from build123d import *

# Parameters (mm, degrees)
SKETCH1_W           = 22
SKETCH1_H           = 26
BOSS_EXTRUDE1_DEPTH = 40
SKETCH2_W           = 18.5
SKETCH2_H           = 22.5
CUT_EXTRUDE1_DEPTH  = 37
CUT_EXTRUDE2_REACH  = 54.536
CUT_EXTRUDE3_DEPTH  = 2
CUT_EXTRUDE4_START  = -1.5
CUT_EXTRUDE4_DEPTH  = 1.5
CUT_EXTRUDE5_REACH  = 54.536
CUT_EXTRUDE6_REACH  = 54.536
SKETCH12_R          = 2.3
BOSS_EXTRUDE2_DEPTH = 7.76
SKETCH14_R          = 1.65
CUT_EXTRUDE9_DEPTH  = 7.76
SKETCH16_R          = 1.65
CUT_EXTRUDE11_DEPTH = 7.76
BOSS_EXTRUDE3_START = 7.76
SKETCH17_R          = 2.3
BOSS_EXTRUDE3_DEPTH = 7.76
CUT_EXTRUDE12_START = -7.76
SKETCH20_R          = 1.65
CUT_EXTRUDE12_DEPTH = 7.76


with BuildPart() as part:
    # Sketch1 → Boss-Extrude1 (new body)
    with BuildSketch(Plane.XY):
        with Locations((11, 13)):
            Rectangle(SKETCH1_W, SKETCH1_H)
    extrude(amount=BOSS_EXTRUDE1_DEPTH)

    # Sketch2 → Cut-Extrude1 (cut)
    with BuildSketch(Plane.XY.offset(40)):
        with Locations((10.75, 13.25)):
            Rectangle(SKETCH2_W, SKETCH2_H)
    extrude(amount=-CUT_EXTRUDE1_DEPTH, mode=Mode.SUBTRACT)

    # Sketch6 → Cut-Extrude2 (cut, up to next)
    with BuildSketch(Plane(origin=(0, 0, 0), x_dir=(-1, 0, 0), z_dir=(0, 0, -1)), mode=Mode.PRIVATE) as cut_extrude2_sk1:
        with BuildLine():
            Line((-15, 22), (-7, 22))
            ThreePointArc((-7, 22), (-3.464466094, 20.535533906), (-2, 17))
            Line((-2, 17), (-2, 9))
            ThreePointArc((-2, 9), (-3.464466094, 5.464466094), (-7, 4))
            Line((-7, 4), (-15, 4))
            ThreePointArc((-15, 4), (-18.535533906, 5.464466094), (-20, 9))
            Line((-20, 9), (-20, 17))
            ThreePointArc((-20, 17), (-18.535533906, 20.535533906), (-15, 22))
        make_face()
    cut_extrude2_tool1 = extrude(cut_extrude2_sk1.sketch, amount=-CUT_EXTRUDE2_REACH, mode=Mode.PRIVATE) & part.part
    add(cut_extrude2_tool1.solids().sort_by_distance((11, 13, 0))[0], mode=Mode.SUBTRACT)

    # Sketch7 → Cut-Extrude3 (cut)
    with BuildSketch(Plane(origin=(22, 0, 0), x_dir=(0, 0, -1), z_dir=(1, 0, 0))):
        with BuildLine():
            Line((-8, 16), (-23, 16))
            Line((-23, 16), (-23, 17))
            ThreePointArc((-23, 17), (-24.464466094, 20.535533906), (-28, 22))
            Line((-28, 22), (-40, 22))
            Line((-40, 22), (-40, 16))
            Line((-40, 16), (-40, 10))
            Line((-40, 10), (-40, 4))
            Line((-40, 4), (-28, 4))
            ThreePointArc((-28, 4), (-24.464466094, 5.464466094), (-23, 9))
            Line((-23, 9), (-23, 10))
            Line((-23, 10), (-8, 10))
            Line((-8, 10), (-8, 16))
        make_face()
    extrude(amount=-CUT_EXTRUDE3_DEPTH, mode=Mode.SUBTRACT)

    # Sketch8 → Cut-Extrude4 (cut)
    with BuildSketch(Plane.ZY.offset(CUT_EXTRUDE4_START)):
        with BuildLine():
            Line((23, 17), (23, 16))
            Line((23, 16), (8, 16))
            Line((8, 16), (8, 10))
            Line((8, 10), (23, 10))
            Line((23, 10), (23, 9))
            ThreePointArc((23, 9), (24.464466094, 5.464466094), (28, 4))
            Line((28, 4), (40, 4))
            Line((40, 4), (40, 22))
            Line((40, 22), (28, 22))
            ThreePointArc((28, 22), (24.464466094, 20.535533906), (23, 17))
        make_face()
    extrude(amount=CUT_EXTRUDE4_DEPTH, mode=Mode.SUBTRACT)

    # Sketch9 → Cut-Extrude5 (cut, up to next)
    with BuildSketch(Plane(origin=(0, 26, 0), x_dir=(1, 0, 0), z_dir=(0, 1, 0)), mode=Mode.PRIVATE) as cut_extrude5_sk1:
        with BuildLine():
            Line((7, -23), (15, -23))
            ThreePointArc((15, -23), (18.535533906, -24.464466094), (20, -28))
            Line((20, -28), (20, -33))
            ThreePointArc((20, -33), (18.535533906, -36.535533906), (15, -38))
            Line((15, -38), (7, -38))
            ThreePointArc((7, -38), (3.464466094, -36.535533906), (2, -33))
            Line((2, -33), (2, -28))
            ThreePointArc((2, -28), (3.464466094, -24.464466094), (7, -23))
        make_face()
    cut_extrude5_tool1 = extrude(cut_extrude5_sk1.sketch, amount=-CUT_EXTRUDE5_REACH, mode=Mode.PRIVATE) & part.part
    # Sketch9 → Cut-Extrude5 (cut, up to next)
    with BuildSketch(Plane(origin=(0, 26, 0), x_dir=(1, 0, 0), z_dir=(0, 1, 0)), mode=Mode.PRIVATE) as cut_extrude5_sk2:
        with BuildLine():
            Line((2, -16.246572976), (2, -8.753427024))
            ThreePointArc((2, -8.753427024), (3.392246541, -5.392246541), (6.753427024, -4))
            Line((6.753427024, -4), (15.246572976, -4))
            ThreePointArc((15.246572976, -4), (18.607753459, -5.392246541), (20, -8.753427024))
            Line((20, -8.753427024), (20, -16.246572976))
            ThreePointArc((20, -16.246572976), (18.607753459, -19.607753459), (15.246572976, -21))
            Line((15.246572976, -21), (6.753427024, -21))
            ThreePointArc((6.753427024, -21), (3.392246541, -19.607753459), (2, -16.246572976))
        make_face()
    cut_extrude5_tool2 = extrude(cut_extrude5_sk2.sketch, amount=-CUT_EXTRUDE5_REACH, mode=Mode.PRIVATE) & part.part
    add(cut_extrude5_tool1.solids().sort_by_distance((11, 26, 30.5))[0], mode=Mode.SUBTRACT)
    add(cut_extrude5_tool2.solids().sort_by_distance((11, 26, 12.5))[0], mode=Mode.SUBTRACT)

    # Sketch11 → Cut-Extrude6 (cut, up to next)
    with BuildSketch(Plane.XZ, mode=Mode.PRIVATE) as cut_extrude6_sk1:
        with BuildLine():
            Line((7, 23), (15, 23))
            ThreePointArc((15, 23), (18.535533906, 24.464466094), (20, 28))
            Line((20, 28), (20, 33))
            ThreePointArc((20, 33), (18.535533906, 36.535533906), (15, 38))
            Line((15, 38), (7, 38))
            ThreePointArc((7, 38), (3.464466094, 36.535533906), (2, 33))
            Line((2, 33), (2, 28))
            ThreePointArc((2, 28), (3.464466094, 24.464466094), (7, 23))
        make_face()
    cut_extrude6_tool1 = extrude(cut_extrude6_sk1.sketch, amount=-CUT_EXTRUDE6_REACH, mode=Mode.PRIVATE) & part.part
    # Sketch11 → Cut-Extrude6 (cut, up to next)
    with BuildSketch(Plane.XZ, mode=Mode.PRIVATE) as cut_extrude6_sk2:
        with BuildLine():
            Line((2, 16), (2, 9))
            ThreePointArc((2, 9), (3.464466094, 5.464466094), (7, 4))
            Line((7, 4), (15, 4))
            ThreePointArc((15, 4), (18.535533906, 5.464466094), (20, 9))
            Line((20, 9), (20, 16))
            ThreePointArc((20, 16), (18.535533906, 19.535533906), (15, 21))
            Line((15, 21), (7, 21))
            ThreePointArc((7, 21), (3.464466094, 19.535533906), (2, 16))
        make_face()
    cut_extrude6_tool2 = extrude(cut_extrude6_sk2.sketch, amount=-CUT_EXTRUDE6_REACH, mode=Mode.PRIVATE) & part.part
    add(cut_extrude6_tool1.solids().sort_by_distance((11, 0, 30.5))[0], mode=Mode.SUBTRACT)
    add(cut_extrude6_tool2.solids().sort_by_distance((11, 0, 12.5))[0], mode=Mode.SUBTRACT)

    # Sketch12 → Boss-Extrude2 (add)
    with BuildSketch(Plane.ZY):
        with Locations(Location((3.63, 5.03, 0), (0, 0, 90))):
            Circle(SKETCH12_R)
        with Locations(Location((19.57, 5.03, 0), (0, 0, 90))):
            Circle(SKETCH12_R)
    extrude(amount=BOSS_EXTRUDE2_DEPTH)

    # Sketch14 → Cut-Extrude9 (cut)
    with BuildSketch(Plane.ZY.offset(7.76)):
        with Locations(Location((3.63, 5.03, 0), (0, 0, 270))):
            Circle(SKETCH14_R)
    extrude(amount=-CUT_EXTRUDE9_DEPTH, mode=Mode.SUBTRACT)

    # Sketch16 → Cut-Extrude11 (cut)
    with BuildSketch(Plane.ZY.offset(7.76)):
        with Locations(Location((19.57, 5.03, 0), (0, 0, 270))):
            Circle(SKETCH16_R)
    extrude(amount=-CUT_EXTRUDE11_DEPTH, mode=Mode.SUBTRACT)

    # Sketch17 → Boss-Extrude3 (add)
    with BuildSketch(Plane(origin=(22, 0, 0), x_dir=(0, 0, -1), z_dir=(1, 0, 0)).offset(BOSS_EXTRUDE3_START)):
        with Locations(Location((-3.63, 5.03, 0), (0, 0, 90))):
            Circle(SKETCH17_R)
        with Locations(Location((-19.57, 5.03, 0), (0, 0, 90))):
            Circle(SKETCH17_R)
    extrude(amount=-BOSS_EXTRUDE3_DEPTH)

    # Sketch20 → Cut-Extrude12 (cut)
    with BuildSketch(Plane(origin=(29.76, 0, 0), x_dir=(0, 0, -1), z_dir=(1, 0, 0)).offset(CUT_EXTRUDE12_START)):
        with Locations(Location((-3.63, 5.03, 0), (0, 0, 270))):
            Circle(SKETCH20_R)
        with Locations(Location((-19.57, 5.03, 0), (0, 0, 270))):
            Circle(SKETCH20_R)
    extrude(amount=CUT_EXTRUDE12_DEPTH, mode=Mode.SUBTRACT)


solid = part.part
For this review, take the finished solid that the model builds, in its own axes (mm). A direction names the side the tool comes from. Give positions to 0.01 mm unless a question says otherwise; leave off trailing zeros. Order: outer loops, then holes, each group sorted by start corner. A loop starts at its lowest first (then second) coordinate and runs counter-clockwise, first axis right, second up. Notation, with made-up numbers: (25.5, 47) - (32.5, 47) arc R22 cw to (32.5, 64) - close; hole circle Ø9 at (69.5, 78). An arc over 180 degrees is marked (long way). Answer as a JSON object with one key per item and string values. Group by question number.
Item 1: Machinability: for faces 5 (the flat face through (11, 1, 38)), 6 (the cylindrical face through (18.645, 25.26, 19.571)), 7 (the flat face through (21, 16, 15)), which of the approach directions +Z, -Z, +X, -X, +Y, -Y give a long, thin tool a straight path to every point of the face, cutting with its end or side? Answer none if there is none.
Item 2: Draft analysis for pull direction Z (two halves, no side actions). For faces 1 (the flat face through (21, 13, 8)), 2 (the cylindrical face through (25.934, 6.266, 21.509)), 3 (the cylindrical face through (-3.83, 6.09, 21.61)), 4 (the flat face through (-7.76, 3, 3)), state which applies: pulls with the +Z half, pulls with the -Z half, needs draft (parallel to the pull), parting line crosses it, or undercut.
Item 3: Wall thickness on line 1 along Z through (x, y) = (25, 5.03); line 2 along X through (y, z) = (7, 14.5); line 3 along Z through (x, y) = (8.5, 24): over which ranges is each line inside the solid? List them lowest first.
Item 4: Take a section at A-A on z = 10. Give the boundary of the cut face in (x, y).
Item 5: Clearance check with flat-ended pins moving along their axes: pin 1 Ø1.6 at (x, y) = (21.5, 12.5) entering from +Z; pin 2 Ø5.5 at (x, z) = (9, 26) entering from +Y; pin 3 Ø2 at (y, z) = (6, 14.5) entering from -X; pin 4 Ø1 at (y, z) = (5, 19.5) entering from +X. State where each tip first meets the part, or that it passes through.
Item 6: Take a section at D-D on z = 32. Give the boundary of the cut face in (x, y).
Item 7: Take a section at C-C on x = 23.5. Give the boundary of the cut face in (y, z).
Item 8: Take a section at B-B on x = 12. Give the boundary of the cut face in (y, z), and give its area (3 significant figures).
Reported:
{
 "1": {"face 5": "+Y, -Y", "face 6": "+Y", "face 7": "+Z, +X, -X"},
 "2": {"face 1": "pulls with the +Z half", "face 2": "undercut", "face 3": "undercut", "face 4": "needs draft"},
 "3": {"line 1": "1.33 to 1.98, 5.28 to 5.93, 17.27 to 17.92, 21.22 to 21.87", "line 2": "0 to 1.5, 20 to 22", "line 3": "0 to 3"},
 "4": {"outline": "(0, 0) - (2, 0) - (2, 2) - (1.5, 2) - (1.5, 10) - (0, 10) - close; (0, 16) - (1.5, 16) - (1.5, 24.5) - (2, 24.5) - (2, 26) - (0, 26) - close; (20, 0) - (22, 0) - (22, 10) - (20, 10) - close; (20, 16) - (22, 16) - (22, 26) - (20, 26) - close"},
 "5": {"pin 1": "z = 8", "pin 2": "through", "pin 3": "x = 0", "pin 4": "x = 22"},
 "6": {"outline": "(0, 0) - (2, 0) - (2, 2) - (1.5, 2) - (1.5, 4) - (0, 4) - close; (0, 22) - (1.5, 22) - (1.5, 24.5) - (2, 24.5) - (2, 26) - (0, 26) - close; (20, 0) - (22, 0) - (22, 4) - (20, 4) - close; (20, 22) - (22, 22) - (22, 26) - (20, 26) - close"},
 "7": {"outline": "circle Ø4.6 at (5.03, 3.63); circle Ø4.6 at (5.03, 19.57); hole circle Ø3.3 at (5.03, 3.63); hole circle Ø3.3 at (5.03, 19.57)"},
 "8": {"outline": "(0, 0) - (4, 0) - (4, 3) - (2, 3) - (2, 4) - (0, 4) - close; (0, 21) - (2, 21) - (2, 23) - (0, 23) - close; (0, 38) - (2, 38) - (2, 40) - (0, 40) - close; (22, 0) - (26, 0) - (26, 4) - (24.5, 4) - (24.5, 3) - (22, 3) - close; (24.5, 21) - (26, 21) - (26, 23) - (24.5, 23) - close; (24.5, 38) - (26, 38) - (26, 40) - (24.5, 40) - close", "area": "41.5 mm^2"}
}
